Source: CAD feature listing. Evaluate the final solid. Frame: model axes, mm. Give positions to 0.01 mm unless a question says otherwise; leave off trailing zeros. Loops run counter-clockwise (first coordinate to the right, second up) from the corner with the lowest first, then second, coordinate; pieces in that order, holes last. Notation, with made-up numbers: (66, 0.25) -> (71, 0.25) arc R14 cw to (71, 16.25) -> close; hole circle Ø7 at (64, 37.5). An arc over 180 degrees is marked (long way). Return JSON: item names as keys, results as strings. Group by question number.
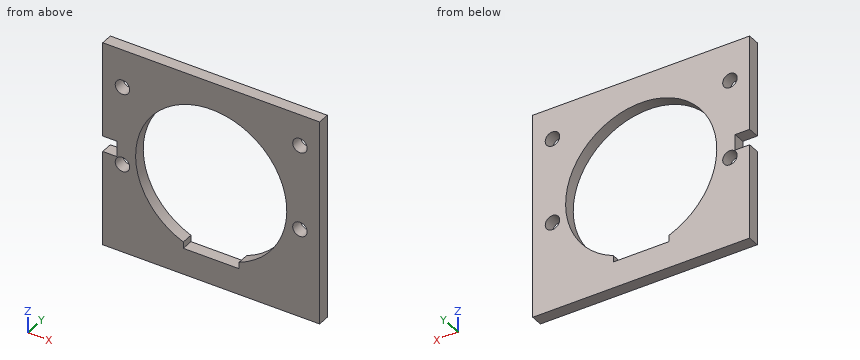
```python
from build123d import *

# Parameters (mm, degrees)
SKETCH5_W      = 41.91
SKETCH5_H      = 39.878
SKETCH5_R      = 1.397
EXTRUDE3_DEPTH = 2.286
SKETCH6_W      = 10.7696
SKETCH6_H      = 20.1676
EXTRUDE4_DEPTH = 3.286
SKETCH7_R      = 14.605
SKETCH7_W      = 2.794
SKETCH7_H      = 3.048
EXTRUDE5_DEPTH = 3.286


with BuildPart() as part:
    # Sketch5 → Extrude3 (new body)
    with BuildSketch(Plane(origin=(0, 0, 0), x_dir=(1, 0, 0), z_dir=(0, 1, 0))):
        with Locations((-20.955, -19.939)):
            Rectangle(SKETCH5_W, SKETCH5_H)
        with Locations((-38.1, -17.272)):
            Circle(SKETCH5_R, mode=Mode.SUBTRACT)
        with Locations((-38.1, -32.512)):
            Circle(SKETCH5_R, mode=Mode.SUBTRACT)
        with Locations((-3.81, -33.782)):
            Circle(SKETCH5_R, mode=Mode.SUBTRACT)
        with Locations((-3.81, -17.272)):
            Circle(SKETCH5_R, mode=Mode.SUBTRACT)
    extrude(amount=EXTRUDE3_DEPTH)

    # Sketch6 → Extrude4 (cut, through all)
    with BuildSketch(Plane(origin=(0, 2.286, 0), x_dir=(-1, 0, 0), z_dir=(0, 1, 0))):
        with Locations((20.955, 15.1892)):
            Rectangle(SKETCH6_W, SKETCH6_H)
    extrude(amount=-EXTRUDE4_DEPTH, mode=Mode.SUBTRACT)

    # Sketch7 → Extrude5 (cut, through all)
    with BuildSketch(Plane.XZ):
        with Locations((-20.955, 19.939)):
            Circle(SKETCH7_R)
        with Locations((-40.513, 19.939)):
            Rectangle(SKETCH7_W, SKETCH7_H)
    extrude(amount=-EXTRUDE5_DEPTH, mode=Mode.SUBTRACT)


solid = part.part
```
1) Cut plane D-D on y = 0.5. Return loops of the section in (x, z) (3 decimals).
2) Cut plane C-C on x = -12.5. Return loops of the section in (y, z), then the cut area to 3 significant figures.
3) Contact query for a flat-ended pin moving along its axis: P1, Ø2.5, axis at x = -3.81, z = 33.782, coming from the -Y side. Output: stop coordinate, or through.
4) Cut plane B-B on z = 22. Return loops of the section in (x, y), then the cut area to 3 significant figures.
5) Material intervals for line 1 (Z direction, x = -3.81, y = 1.7) (3 decimals); line 2 (Z direction, x = -3.5, y = 1.5); line 3 (X direction, y = 1.85, z = 6), sorted ascending.
6) Cut plane A-A on x = -38.1. Return loops of the section in (y, z) (3 decimals).
Calculated:
{
 "1": {"outline": "(-41.91, 0) -> (0, 0) -> (0, 39.878) -> (-41.91, 39.878) -> (-41.91, 21.463) -> (-39.116, 21.463) -> (-39.116, 18.415) -> (-41.91, 18.415) -> close; hole circle Ø2.794 at (-38.1, 17.272); hole circle Ø2.794 at (-38.1, 32.512); hole (-26.34, 5.105) -> (-15.57, 5.105) -> (-15.57, 6.363) arc R14.605 ccw (long way) to (-26.34, 6.363) -> close; hole circle Ø2.794 at (-3.81, 17.272); hole circle Ø2.794 at (-3.81, 33.782)"},
 "2": {"outline": "(0, 0) -> (2.29, 0) -> (2.29, 8.03) -> (0, 8.03) -> close; (0, 31.85) -> (2.29, 31.85) -> (2.29, 39.88) -> (0, 39.88) -> close", "area": "36.7 mm2"},
 "3": {"P1": "through"},
 "4": {"outline": "(-41.91, 0) -> (-35.41, 0) -> (-35.41, 2.29) -> (-41.91, 2.29) -> close; (-6.5, 0) -> (0, 0) -> (0, 2.29) -> (-6.5, 2.29) -> close", "area": "29.7 mm2"},
 "5": {"line 1": "0 to 15.875, 18.669 to 32.385, 35.179 to 39.878", "line 2": "0 to 15.91, 18.63 to 32.42, 35.14 to 39.88", "line 3": "-41.91 to -26.34, -15.57 to 0"},
 "6": {"outline": "(0, 0) -> (2.286, 0) -> (2.286, 15.875) -> (0, 15.875) -> close; (0, 18.669) -> (2.286, 18.669) -> (2.286, 31.115) -> (0, 31.115) -> close; (0, 33.909) -> (2.286, 33.909) -> (2.286, 39.878) -> (0, 39.878) -> close"}
}
